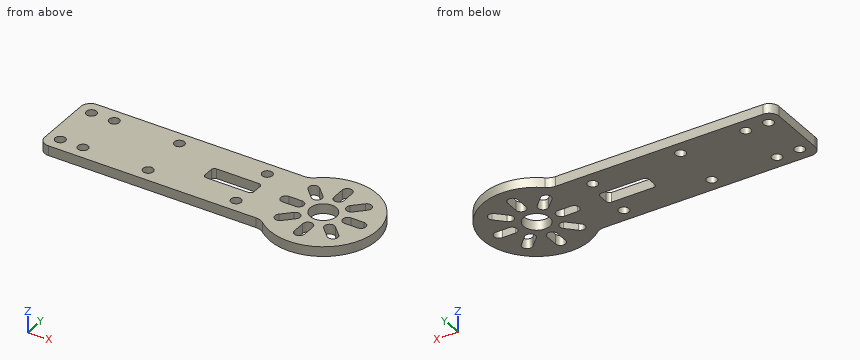
```python
from build123d import *

# Parameters (mm, degrees)
SKETCH_1_R      = 4
SKETCH_1_R_2    = 1.56
EXTRUDE_3_DEPTH = 3


with BuildPart() as part:
    # 草图1 → 凸台-拉伸3 (new body)
    with BuildSketch(Plane.XY):
        with BuildLine():
            Line((-13.220699864, 11.66726189), (-77, 11.66726189))
            ThreePointArc((-77, 11.66726189), (-79.121320344, 10.788582233), (-80, 8.66726189))
            Line((-80, 8.66726189), (-80, -8.66726189))
            ThreePointArc((-80, -8.66726189), (-79.121320344, -10.788582233), (-77, -11.66726189))
            Line((-77, -11.66726189), (-13.220699864, -11.66726189))
            ThreePointArc((-13.220699864, -11.66726189), (-11.847402161, -11.910394389), (-10.64105111, -12.610235179))
            ThreePointArc((-10.64105111, -12.610235179), (16.5, 0), (-10.64105111, 12.610235179))
            ThreePointArc((-10.64105111, 12.610235179), (-11.847402161, 11.910394389), (-13.220699864, 11.66726189))
        make_face()
        Circle(SKETCH_1_R, mode=Mode.SUBTRACT)
        with Locations((-76, 7.5)):
            Circle(SKETCH_1_R_2, mode=Mode.SUBTRACT)
        with Locations((-76, -7.5)):
            Circle(SKETCH_1_R_2, mode=Mode.SUBTRACT)
        with Locations((-69, 7.5)):
            Circle(SKETCH_1_R_2, mode=Mode.SUBTRACT)
        with Locations((-69, -7.5)):
            Circle(SKETCH_1_R_2, mode=Mode.SUBTRACT)
        with Locations((-49, 7.5)):
            Circle(SKETCH_1_R_2, mode=Mode.SUBTRACT)
        with Locations((-49, -7.5)):
            Circle(SKETCH_1_R_2, mode=Mode.SUBTRACT)
        with Locations((-22, 7.5)):
            Circle(SKETCH_1_R_2, mode=Mode.SUBTRACT)
        with Locations((-22, -7.5)):
            Circle(SKETCH_1_R_2, mode=Mode.SUBTRACT)
        with BuildLine():
            Line((-11.525767243, 1.55), (-7.525767243, 1.55))
            ThreePointArc((-7.525767243, 1.55), (-5.975767243, 0), (-7.525767243, -1.55))
            Line((-7.525767243, -1.55), (-11.525767243, -1.55))
            ThreePointArc((-11.525767243, -1.55), (-13.075767243, 0), (-11.525767243, 1.55))
        make_face(mode=Mode.SUBTRACT)
        with BuildLine():
            Line((11.525767243, 1.55), (7.525767243, 1.55))
            ThreePointArc((7.525767243, 1.55), (5.975767243, 0), (7.525767243, -1.55))
            Line((7.525767243, -1.55), (11.525767243, -1.55))
            ThreePointArc((11.525767243, -1.55), (13.075767243, 0), (11.525767243, 1.55))
        make_face(mode=Mode.SUBTRACT)
        with BuildLine():
            Line((-7.017492281, 9.209523303), (-4.189065156, 6.381096178))
            ThreePointArc((-4.189065156, 6.381096178), (-4.189065156, 4.189065156), (-6.381096178, 4.189065156))
            Line((-6.381096178, 4.189065156), (-9.209523303, 7.017492281))
            ThreePointArc((-9.209523303, 7.017492281), (-9.209523303, 9.209523303), (-7.017492281, 9.209523303))
        make_face(mode=Mode.SUBTRACT)
        with BuildLine():
            Line((1.55, -11.474232757), (1.55, -7.474232757))
            ThreePointArc((1.55, -7.474232757), (0, -5.924232757), (-1.55, -7.474232757))
            Line((-1.55, -7.474232757), (-1.55, -11.474232757))
            ThreePointArc((-1.55, -11.474232757), (0, -13.024232757), (1.55, -11.474232757))
        make_face(mode=Mode.SUBTRACT)
        with BuildLine():
            Line((1.55, 11.525767243), (1.55, 7.525767243))
            ThreePointArc((1.55, 7.525767243), (0, 5.975767243), (-1.55, 7.525767243))
            Line((-1.55, 7.525767243), (-1.55, 11.525767243))
            ThreePointArc((-1.55, 11.525767243), (0, 13.075767243), (1.55, 11.525767243))
        make_face(mode=Mode.SUBTRACT)
        with BuildLine():
            Line((7.017492281, 9.209523303), (4.189065156, 6.381096178))
            ThreePointArc((4.189065156, 6.381096178), (4.189065156, 4.189065156), (6.381096178, 4.189065156))
            Line((6.381096178, 4.189065156), (9.209523303, 7.017492281))
            ThreePointArc((9.209523303, 7.017492281), (9.209523303, 9.209523303), (7.017492281, 9.209523303))
        make_face(mode=Mode.SUBTRACT)
        with BuildLine():
            Line((-7.017492281, -9.209523303), (-4.189065156, -6.381096178))
            ThreePointArc((-4.189065156, -6.381096178), (-4.189065156, -4.189065156), (-6.381096178, -4.189065156))
            Line((-6.381096178, -4.189065156), (-9.209523303, -7.017492281))
            ThreePointArc((-9.209523303, -7.017492281), (-9.209523303, -9.209523303), (-7.017492281, -9.209523303))
        make_face(mode=Mode.SUBTRACT)
        with BuildLine():
            Line((7.017492281, -9.209523303), (4.189065156, -6.381096178))
            ThreePointArc((4.189065156, -6.381096178), (4.189065156, -4.189065156), (6.381096178, -4.189065156))
            Line((6.381096178, -4.189065156), (9.209523303, -7.017492281))
            ThreePointArc((9.209523303, -7.017492281), (9.209523303, -9.209523303), (7.017492281, -9.209523303))
        make_face(mode=Mode.SUBTRACT)
        with BuildLine():
            Line((-34.37331228, 2.5), (-21.37331228, 2.5))
            ThreePointArc((-21.37331228, 2.5), (-20.666205499, 2.207106781), (-20.37331228, 1.5))
            Line((-20.37331228, 1.5), (-20.37331228, -1.5))
            ThreePointArc((-20.37331228, -1.5), (-20.666205499, -2.207106781), (-21.37331228, -2.5))
            Line((-21.37331228, -2.5), (-34.37331228, -2.5))
            ThreePointArc((-34.37331228, -2.5), (-35.080419062, -2.207106781), (-35.37331228, -1.5))
            Line((-35.37331228, -1.5), (-35.37331228, 1.5))
            ThreePointArc((-35.37331228, 1.5), (-35.080419062, 2.207106781), (-34.37331228, 2.5))
        make_face(mode=Mode.SUBTRACT)
    extrude(amount=EXTRUDE_3_DEPTH)


solid = part.part
```
Geometry: final body of the model. Coordinates: model frame, mm. Round coordinates to 2 decimals unless told otherwise and drop trailing zeros. Order: outer loops, then holes, each group sorted by start corner. A loop starts at its lowest first (then second) coordinate and runs counter-clockwise, first axis right, second up. Notation, with made-up numbers: M 21,-14 L 79,-14 A9 ccw 79,-7 Z; hole C 12.5,61.5 d5. An arc over 180 degrees is marked long. Use one line per item in the form item = value. Start each with the question number.
Q1. Cut plane A-A (x = 0). Return loops of the section in (y, z).
Q2. Cut plane C-C (x = -69). Return loops of the section in (y, z), and give its area (3 significant figures).
Q3. Cut plane D-D (x = -29). Return loops of the section in (y, z), and give its area (3 significant figures).
Q4. Pin query (flat end, axial travel): pin 1 Ø1.5 at (x, z) = (-28, 1) entering from +Y; pin 2 Ø1 at (x, z) = (-21.5, 2) entering from -Y; pin 3 Ø1.5 at (x, z) = (10.5, 2) entering from +Y. Return the tip coordinate at first contact, or that it passes through.
Q5. Cut plane B-B (y = 0). Return loops of the section in (x, z).
Q6. Material intervals for line 1 (Y direction, x = -69, z = 1.1); line 2 (Y direction, x = -22, z = 2.3); line 3 (Y direction, x = -31, z = 1.7), sorted ascending. Write a range as [from, to].
Geometry results:
q1.outline = M -16.5,0 L -13.02,0 L -13.02,3 L -16.5,3 Z; M -5.92,0 L -4,0 L -4,3 L -5.92,3 Z; M 4,0 L 5.98,0 L 5.98,3 L 4,3 Z; M 13.08,0 L 16.5,0 L 16.5,3 L 13.08,3 Z
q2.outline = M -11.67,0 L -9.06,0 L -9.06,3 L -11.67,3 Z; M -5.94,0 L 5.94,0 L 5.94,3 L -5.94,3 Z; M 9.06,0 L 11.67,0 L 11.67,3 L 9.06,3 Z
q2.area = 51.3 mm^2
q3.outline = M -11.67,0 L -2.5,0 L -2.5,3 L -11.67,3 Z; M 2.5,0 L 11.67,0 L 11.67,3 L 2.5,3 Z
q3.area = 55.0 mm^2
q4.pin_1 = 11.67
q4.pin_2 = -11.67
q4.pin_3 = 13.31
q5.outline = M -80,0 L -35.37,0 L -35.37,3 L -80,3 Z; M -20.37,0 L -13.08,0 L -13.08,3 L -20.37,3 Z; M -5.98,0 L -4,0 L -4,3 L -5.98,3 Z; M 4,0 L 5.98,0 L 5.98,3 L 4,3 Z; M 13.08,0 L 16.5,0 L 16.5,3 L 13.08,3 Z
q6.line_1 = [-11.67, -9.06], [-5.94, 5.94], [9.06, 11.67]
q6.line_2 = [-11.67, -9.06], [-5.94, -2.5], [2.5, 5.94], [9.06, 11.67]
q6.line_3 = [-11.67, -2.5], [2.5, 11.67]
